```python
from build123d import *

# Parameters (mm, degrees)
EXTRUDE_1_DEPTH          = 62.115
EXTRUDE_START            = -62.995
SKETCH_2_W               = 10
SKETCH_2_H               = 28
EXTRUDE_2_DEPTH          = 62.995
CUT_EXTRUDE_1_DEPTH      = 10
SKETCH_4_R               = 1.6
CUT_EXTRUDE_2_DEPTH      = 3
CUT_EXTRUDE_3_DEPTH      = 10
SKETCH_6_R               = 5.6
SKETCH_6_R_2             = 2.6
EXTRUDE_3_DEPTH          = 14.433757
CUT_EXTRUDE_4_DEPTH      = 20
CUT_EXTRUDE_5_DEPTH      = 10
CUT_EXTRUDE_5_DEPTH_BACK = 8
SKETCH_7_R               = 3.95
CUT_EXTRUDE_START        = 10
CUT_EXTRUDE_6_DEPTH      = 10
CHAMFER_1_SIZE           = 1
CUT_EXTRUDE_7_DEPTH      = 10
CUT_EXTRUDE_8_DEPTH      = 143.906491892
EXTRUDE_START_2          = 1.73
SKETCH_10_R              = 2.6
EXTRUDE_4_DEPTH          = 1.73


with BuildPart() as part:
    # Эскиз1 → Бобышка-Вытянуть1 (new, symmetric)
    with BuildSketch(Plane.XY):
        Polygon((-62.995, 0), (-45.262949192, 0), (-30.829192463, 25), (0, 25), (0, 28), (-32.56124327, 28), (-46.995, 3), (-62.995, 3), align=None)
    extrude(amount=EXTRUDE_1_DEPTH, both=True)

    # Эскиз2 → Бобышка-Вытянуть2 (add)
    with BuildSketch(Plane(origin=(0, 0, 0), x_dir=(0, 0, -1), z_dir=(1, 0, 0)).offset(EXTRUDE_START)):
        with Locations((0, 14)):
            Rectangle(SKETCH_2_W, SKETCH_2_H)
    extrude(amount=EXTRUDE_2_DEPTH)

    # Эскиз3 → Вырез-Вытянуть1 (cut)
    with BuildSketch(Plane.XY.offset(5)):
        Polygon((0, 25), (0, 0), (-45.262949192, 0), (-30.829192463, 25), align=None)
    extrude(amount=-CUT_EXTRUDE_1_DEPTH, mode=Mode.SUBTRACT)

    # Эскиз4 → Вырез-Вытянуть2 (cut)
    with BuildSketch(Plane.XZ):
        with Locations(Location((-54.995, 0, 0), (0, 0, 270))):
            Circle(SKETCH_4_R)
        with Locations(Location((-54.995, -15.52875, 0), (0, 0, 270))):
            Circle(SKETCH_4_R)
        with Locations(Location((-54.995, -31.0575, 0), (0, 0, 270))):
            Circle(SKETCH_4_R)
        with Locations(Location((-54.995, -46.58625, 0), (0, 0, 270))):
            Circle(SKETCH_4_R)
        with Locations(Location((-54.995, 46.58625, 0), (0, 0, 90))):
            Circle(SKETCH_4_R)
        with Locations(Location((-54.995, 31.0575, 0), (0, 0, 90))):
            Circle(SKETCH_4_R)
        with Locations(Location((-54.995, 15.52875, 0), (0, 0, 90))):
            Circle(SKETCH_4_R)
    extrude(amount=-CUT_EXTRUDE_2_DEPTH, mode=Mode.SUBTRACT)

    # Эскиз5 → Вырез-Вытянуть3 (cut)
    with BuildSketch(Plane(origin=(0, 0, -5), x_dir=(-1, 0, 0), z_dir=(0, 0, -1))):
        Polygon((46.995, 3), (62.995, 3), (62.995, 28), (46.995, 28), (46.995, 24.7), (37.598624369, 19.275), align=None)
    extrude(amount=-CUT_EXTRUDE_3_DEPTH, mode=Mode.SUBTRACT)

    # Эскиз6 → Бобышка-Вытянуть3 (add)
    with BuildSketch(Plane.ZY.offset(46.995)):
        with Locations((0, 26.35)):
            Circle(SKETCH_6_R)
        with Locations((0, 26.35)):
            Circle(SKETCH_6_R_2, mode=Mode.SUBTRACT)
    extrude(amount=-EXTRUDE_3_DEPTH)

    # Эскиз6<2> → Вырез-Вытянуть4 (cut)
    with BuildSketch(Plane.ZY.offset(46.995)):
        with BuildLine():
            Line((-2.00935313, 28), (0, 28))
            Line((0, 28), (2.00935313, 28))
            ThreePointArc((2.00935313, 28), (0, 28.95), (-2.00935313, 28))
        make_face()
        with BuildLine():
            Line((-2.00935313, 24.7), (0, 24.7))
            Line((0, 24.7), (0, 28))
            Line((0, 28), (-2.00935313, 28))
            ThreePointArc((-2.00935313, 28), (-2.6, 26.35), (-2.00935313, 24.7))
        make_face()
        with BuildLine():
            Line((0, 28), (0, 24.7))
            Line((0, 24.7), (2.00935313, 24.7))
            ThreePointArc((2.00935313, 24.7), (2.447888696, 25.473734668), (2.6, 26.35))
            ThreePointArc((2.6, 26.35), (2.447888696, 27.226265332), (2.00935313, 28))
            Line((2.00935313, 28), (0, 28))
        make_face()
        with BuildLine():
            Line((2.00935313, 24.7), (0, 24.7))
            Line((0, 24.7), (-2.00935313, 24.7))
            ThreePointArc((-2.00935313, 24.7), (0, 23.75), (2.00935313, 24.7))
        make_face()
    extrude(amount=-CUT_EXTRUDE_4_DEPTH, mode=Mode.SUBTRACT)

    # Эскиз7 → Вырез-Вытянуть5 (cut, two sides: drawn at the far end of the back side and taken through both)
    with BuildSketch(Plane(origin=(-32.56124327, 0, 0), x_dir=(0, 0, -1), z_dir=(1, 0, 0)).offset(-CUT_EXTRUDE_5_DEPTH_BACK)):
        with Locations(Location((0, 26.35, 0), (0, 0, 199.984879971))):
            Circle(SKETCH_7_R)
    extrude(amount=CUT_EXTRUDE_5_DEPTH + CUT_EXTRUDE_5_DEPTH_BACK, mode=Mode.SUBTRACT)

    # Эскиз8 → Вырез-Вытянуть6 (cut)
    with BuildSketch(Plane.ZY.offset(22.56124327).offset(CUT_EXTRUDE_START)):
        with BuildLine():
            Line((-3.95, 26.35), (-3.95, 28))
            Line((-3.95, 28), (3.95, 28))
            Line((3.95, 28), (3.95, 26.35))
            ThreePointArc((3.95, 26.35), (3.890081094, 25.664602977), (3.712142239, 25))
            Line((3.712142239, 25), (-3.712142239, 25))
            ThreePointArc((-3.712142239, 25), (-3.890081094, 25.664602977), (-3.95, 26.35))
        make_face()
    extrude(amount=-CUT_EXTRUDE_6_DEPTH, mode=Mode.SUBTRACT)

    # Фаска1
    chamfer_1_edges = [part.edges().sort_by_distance(p)[0] for p in [
        (-27.56124327, 28, 3.95),
        (-27.56124327, 28, -3.95),
    ]]
    chamfer(chamfer_1_edges, length=CHAMFER_1_SIZE)

    # Эскиз3<2> → Вырез-Вытянуть7 (cut)
    with BuildSketch(Plane.XY.offset(5)):
        Polygon((0, 25), (0, 0), (-45.262949192, 0), (-30.829192463, 25), align=None)
    extrude(amount=-CUT_EXTRUDE_7_DEPTH, mode=Mode.SUBTRACT)

    # Эскиз9 → Вырез-Вытянуть8 (cut, through all)
    with BuildSketch(Plane.XY.offset(62.115)):
        Polygon((-45.262949192, 6), (-45.262949192, 31.95), (-62.995, 31.95), (-62.995, 3), (-46.995, 3), align=None)
    extrude(amount=-CUT_EXTRUDE_8_DEPTH, mode=Mode.SUBTRACT)

    # Эскиз10 → Бобышка-Вытянуть4 (add)
    with BuildSketch(Plane.ZY.offset(45.262949192).offset(EXTRUDE_START_2)):
        with BuildLine():
            Line((-5, 23.828095957), (-4.93330518, 23.7))
            ThreePointArc((-4.93330518, 23.7), (0, 20.75), (4.93330518, 23.7))
            Line((4.93330518, 23.7), (5, 23.828095957))
            ThreePointArc((5, 23.828095957), (0, 31.95), (-5, 23.828095957))
        make_face()
        with Locations((0, 26.35)):
            Circle(SKETCH_10_R, mode=Mode.SUBTRACT)
    extrude(amount=-EXTRUDE_4_DEPTH)

    # Зеркальное отражение1: part across plane


with BuildPart() as part_1:
    add(part.part)
    add(part.part.mirror(Plane(origin=(0, 25, 62.115), x_dir=(0, 0, 1), z_dir=(-1, 0, 0))))


solid = part_1.part
```
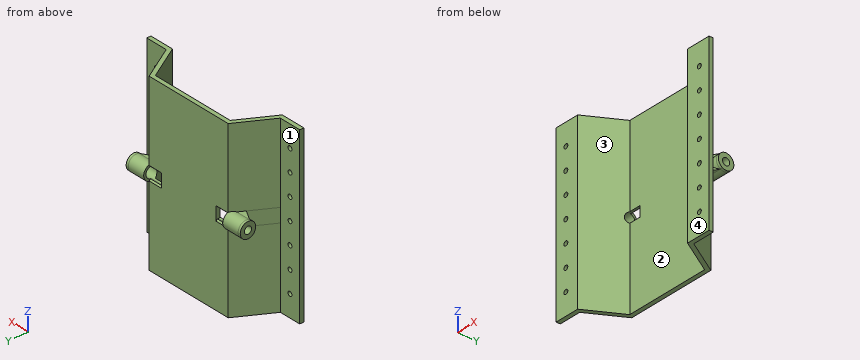
Verification items for the finished model (mm, model axes). Face numbers are marked on the shaded views. A direction names the side the tool comes from. Coordinates: 2 decimals unless noted, no trailing zeros. Loops run counter-clockwise (first coordinate to the right, second up) from the corner with the lowest first, then second, coordinate; pieces in that order, holes last. Notation, with made-up numbers: (53, 48.25) - (66, 48.25) arc R31 ccw to (66, 78.25) - close; hole circle Ø11 at (74, 50.25). An arc over 180 degrees is marked (long way). Put each result on its own line as item: value.
Item 1: Draft check along X on the marked faces 1 and 2. Enter one of: pulls with the +X half, pulls with the -X half, needs draft (parallel to the pull), parting line crosses it, or undercut.
Conclusion:
face 1: needs draft
face 2: undercut
Item 2: Section check B-B (z = -43). Enter the section's corners in (x, y) (3 decimals), then the cut area to 3 significant figures.
Conclusion:
outline: (-62.995, 0) - (-45.263, 0) - (-30.829, 25) - (30.829, 25) - (45.263, 0) - (62.995, 0) - (62.995, 3) - (46.995, 3) - (32.561, 28) - (-32.561, 28) - (-46.995, 3) - (-62.995, 3) - close
area: 465 mm2
Item 3: Set-up check for the marked faces 3 and 4: record each of +Z, -Z, +X, -X, +Y, -Y from which the full face is reachable in a straight line by a thin tool's end or side.
Conclusion:
face 3: +Z, -Z, -Y
face 4: +Z, -Z, +X, -X, -Y
Item 4: Scan lines: line 1 along Y through (x, z) = (-30, 30.5); line 2 along X through (y, z) = (5.5, -23.5); line 3 along X through (y, z) = (15, -16.5). Record each from-to range of solid material in increasing order.
Conclusion:
line 1: y = 25 to 28
line 2: x = -45.55 to -42.09, 42.09 to 45.55
line 3: x = -40.07 to -36.6, 36.6 to 40.07
Item 5: Gauge pin test, flat ends, axial feed: pin 1 Ø10 at (y, z) = (11, 14) entering from +X; pin 2 Ø2.5 at (y, z) = (25.5, -1) entering from -X; pin 3 Ø3 at (x, z) = (-13, -35) entering from -Y. Record the tip position at first contact, or that the pin passes through.
Conclusion:
pin 1: stops at x = 45.26
pin 2: stops at x = -22.56
pin 3: stops at y = 25
Item 6: Section check C-C (y = 17). Enter the section's corners in (x, z) (3 decimals), then the cut area to 3 significant figures.
Conclusion:
outline: (-38.912, -62.115) - (-35.448, -62.115) - (-35.448, 62.115) - (-38.912, 62.115) - close; (35.448, -62.115) - (38.912, -62.115) - (38.912, 62.115) - (35.448, 62.115) - close
area: 861 mm2
